Here's the drawing with two shaded views (mm, measured from the low corner). I have some questions. A direction names the side the tool comes from. Give positions to 0.01 mm unless a question says otherwise; leave off trailing zeros. Write each loop counter-clockwise with the first axis right and the second up, starting at its lowest first coordinate (ties: lowest second). Pieces come first, ordered by that corner, then holes. Notation, with made-up numbers: (24.25, 29.25) -> (50.25, 29.25) arc R7 ccw to (50.25, 41.25) -> close; hole circle Ø1 at (33, 80.25). An arc over 180 degrees is marked (long way). One line per question, with ' | ' between items.
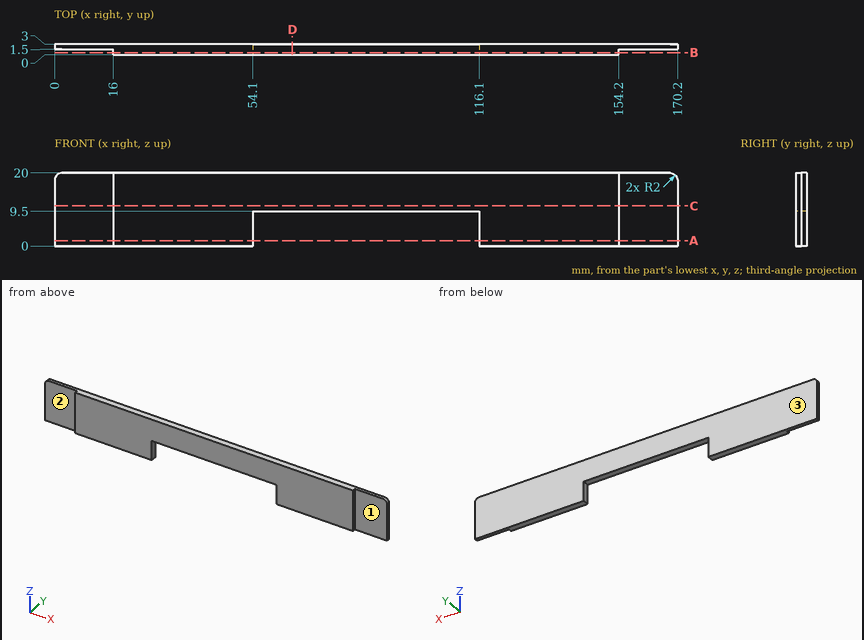
Q1. On a 3-axis mill with a long thin cutter (end or side, diameter ignored), from which of +Z, -Z, +X, -X, +Y, -Y can I reach the whole of each face in a straight line? I mean the marked faces 1, 2 and 3. Say none if no direction works.
Answer below:
face 1: +Z, -Z, +X, -Y | face 2: +Z, -Z, -X, -Y | face 3: +Z, -Z, +X, -X, +Y
Q2. Imagine slicing it at A-A on z = 1.5. Please give me the cut outline in (x, y), and give its area (3 significant figures).
Answer below:
outline: (0, 1.5) -> (16, 1.5) -> (16, 0) -> (54.1, 0) -> (54.1, 3) -> (0, 3) -> close; (116.1, 0) -> (154.2, 0) -> (154.2, 1.5) -> (170.2, 1.5) -> (170.2, 3) -> (116.1, 3) -> close | area: 277 mm^2
Q3. Imagine slicing it at C-C on z = 11. Please give me the cut outline in (x, y).
Answer below:
outline: (0, 1.5) -> (16, 1.5) -> (16, 0) -> (154.2, 0) -> (154.2, 1.5) -> (170.2, 1.5) -> (170.2, 3) -> (0, 3) -> close
Q4. Imagine slicing it at D-D on x = 65. Please give me the cut outline in (y, z).
Answer below:
outline: (0, 9.5) -> (3, 9.5) -> (3, 20) -> (0, 20) -> close
Q5. If I drill on line 1 along X through (y, z) = (2, 6.25); line 2 along X through (y, z) = (0.2, 8.75); line 3 along Z through (x, y) = (93, 1.4), over which ranges is the centre line in solid material (lowest first)?
Answer below:
line 1: x = 0 to 54.1, 116.1 to 170.2 | line 2: x = 16 to 54.1, 116.1 to 154.2 | line 3: z = 9.5 to 20
Q6. Imagine slicing it at B-B on y = 0.65. Please give me the cut outline in (x, z).
Answer below:
outline: (16, 0) -> (54.1, 0) -> (54.1, 9.5) -> (116.1, 9.5) -> (116.1, 0) -> (154.2, 0) -> (154.2, 20) -> (16, 20) -> close
Q7. Will these pins go through, and if not, where does the flat tip stop? pin 1 (5 mm diameter, centred on x = 166, z = 6.5, fed in from -Y); pin 2 (0.8 mm diameter, centred on y = 0.5, z = 7.5, fed in from +X); pin 3 (1.5 mm diameter, centred on x = 80, y = 2, fed in from -Z).
Answer below:
pin 1: stops at y = 1.5 | pin 2: stops at x = 154.2 | pin 3: stops at z = 9.5
